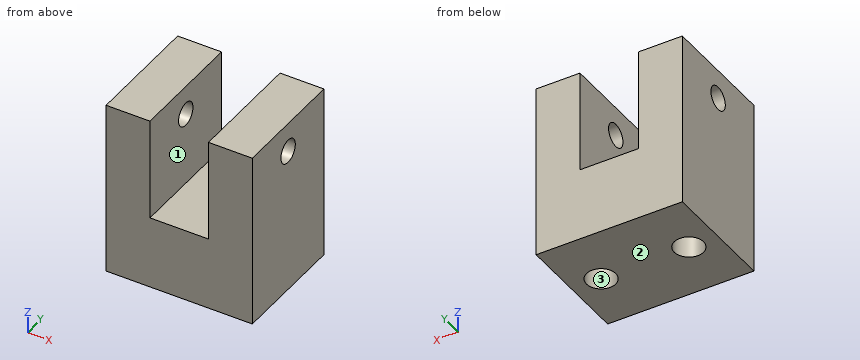
```python
from build123d import *

# Parameters (mm, degrees)
SKETCH1_W                       = 31.75
SKETCH1_H                       = 25.4
BOSS_EXTRUDE1_DEPTH             = 38.1
F_1_4_0_25_DIAMETER_HOLE1_D     = 6.35
F_1_4_0_25_DIAMETER_HOLE1_DEPTH = 12.7
F_1_4_0_25_DIAMETER_HOLE1_TIP   = 1.907732465
SKETCH5_W                       = 12.7
SKETCH5_H                       = 22.225
CUT_EXTRUDE2_DEPTH              = 26.4
F_10_CLEARANCE_HOLE1_D          = 5.1054


with BuildPart() as part:
    # Sketch1 → Boss-Extrude1 (new body)
    with BuildSketch(Plane.XY):
        with Locations((15.875, 12.7)):
            Rectangle(SKETCH1_W, SKETCH1_H)
    extrude(amount=BOSS_EXTRUDE1_DEPTH)

    # 1/4 (0.25) Diameter Hole1
    with Locations(Plane(origin=(0, 0, 0), x_dir=(-1, 0, 0), z_dir=(0, 0, -1))):
        with Locations((-25.4, 12.7), (-6.35, 12.7)):
            Hole(F_1_4_0_25_DIAMETER_HOLE1_D / 2, depth=F_1_4_0_25_DIAMETER_HOLE1_DEPTH)
            with Locations((0, 0, -(F_1_4_0_25_DIAMETER_HOLE1_DEPTH + F_1_4_0_25_DIAMETER_HOLE1_TIP / 2))):  # 118° drill point
                Cone(0, F_1_4_0_25_DIAMETER_HOLE1_D / 2, F_1_4_0_25_DIAMETER_HOLE1_TIP, mode=Mode.SUBTRACT)

    # Sketch5 → Cut-Extrude2 (cut, through all)
    with BuildSketch(Plane(origin=(0, 25.4, 0), x_dir=(1, 0, 0), z_dir=(0, 1, 0))):
        with Locations((15.875, -26.9875)):
            Rectangle(SKETCH5_W, SKETCH5_H)
    extrude(amount=-CUT_EXTRUDE2_DEPTH, mode=Mode.SUBTRACT)

    # #10 Clearance Hole1 (through all)
    with Locations(Plane(origin=(31.75, 0, 0), x_dir=(0, 0, -1), z_dir=(1, 0, 0))):
        with Locations((-31.75, 12.7)):
            Hole(F_10_CLEARANCE_HOLE1_D / 2)


solid = part.part
```
For this review, take the finished solid that the model builds, in its own axes (mm). Face numbers are marked on the shaded views. A direction names the side the tool comes from. Give positions to 0.01 mm unless a question says otherwise; leave off trailing zeros. Loops run counter-clockwise (first coordinate to the right, second up) from the corner with the lowest first, then second, coordinate; pieces in that order, holes last. Notation, with made-up numbers: M 68,33.5 L 84,33.5 A23 ccw 84,67.5 Z; hole C 38.25,37 d4. An arc over 180 degrees is marked long. One line per item, written item: value. Start each with the question number.
Q1. For L1, parallel to X at y = 12.7, z = 2.5 (3 decimals); L2, parallel to X at y = 17.5, z = 32.5 (3 decimals); L3, parallel to Y at x = 6.35, z = 5.5 (3 decimals), list the stretches that pass through material, from the lowest coordinate up.
Q2. Add section A-A (z = 31.75). Give the boundary of the cut face in (x, y) (3 decimals).
Q3. Clearance check with flat-ended pins moving along their axes: pin 1 Ø6.5 at (x, y) = (14, 7) entering from +Z (3 decimals); pin 2 Ø10 at (y, z) = (11.5, 26.5) entering from -X. State where each tip first meets the part, or that it passes through.
Q4. Add section C-C (z = 27.5). Give the boundary of the cut face in (x, y) (3 decimals).
Q5. Add section B-B (x = 29.5). Give the boundary of the cut face in (y, z), and give its area (3 significant figures).
Q6. Add section D-D (y = 21.75). Give the boundary of the cut face in (x, z) (3 decimals), and give its area (3 significant figures).
Q7. Machinability: for the marked faces 1, 2 and 3, which of the approach directions +Z, -Z, +X, -X, +Y, -Y give a long, thin tool a straight path to every point of the face, cutting with its end or side? Answer none if there is none.
Reply:
1. L1: 0 to 3.175, 9.525 to 22.225, 28.575 to 31.75
1. L2: 0 to 9.525, 22.225 to 31.75
1. L3: 0 to 9.525, 15.875 to 25.4
2. outline: M 0,0 L 9.525,0 L 9.525,10.147 L 0,10.147 Z; M 0,15.253 L 9.525,15.253 L 9.525,25.4 L 0,25.4 Z; M 22.225,0 L 31.75,0 L 31.75,10.147 L 22.225,10.147 Z; M 22.225,15.253 L 31.75,15.253 L 31.75,25.4 L 22.225,25.4 Z
3. pin 1: z = 15.875
3. pin 2: x = 0
4. outline: M 0,0 L 9.525,0 L 9.525,25.4 L 0,25.4 Z; M 22.225,0 L 31.75,0 L 31.75,25.4 L 22.225,25.4 Z
5. outline: M 0,0 L 25.4,0 L 25.4,38.1 L 0,38.1 Z; hole C 12.7,31.75 d5.11
5. area: 947 mm²
6. outline: M 0,0 L 31.75,0 L 31.75,38.1 L 22.225,38.1 L 22.225,15.875 L 9.525,15.875 L 9.525,38.1 L 0,38.1 Z
6. area: 927 mm²
7. face 1: +Z, +Y, -Y
7. face 2: -Z, +X, -X, +Y, -Y
7. face 3: -Z
